from build123d import *

# Parameters (mm, degrees)
ESQUISSE1_W        = 1810
ESQUISSE1_H        = 1810
BOSS_EXTRU_1_DEPTH = 10
ESQUISSE2_W        = 1810
ESQUISSE2_H        = 1810
ESQUISSE2_W_2      = 1750
ESQUISSE2_H_2      = 1750
BOSS_EXTRU_2_DEPTH = 50
ESQUISSE3_W        = 1750
ESQUISSE3_H        = 30
BOSS_EXTRU_3_DEPTH = 50
ESQUISSE4_W        = 30
ESQUISSE4_H        = 1750
BOSS_EXTRU_4_DEPTH = 50
ESQUISSE5_W        = 1810
ESQUISSE5_H        = 1810
ESQUISSE5_W_2      = 1786
ESQUISSE5_H_2      = 1786
BOSS_EXTRU_5_DEPTH = 50


with BuildPart() as part:
    # Esquisse1 → Boss.-Extru.1 (new body)
    with BuildSketch(Plane(origin=(0, 0, 0), x_dir=(1, 0, 0), z_dir=(0, 1, 0))):
        Rectangle(ESQUISSE1_W, ESQUISSE1_H)
    extrude(amount=BOSS_EXTRU_1_DEPTH)

    # Esquisse2 → Boss.-Extru.2 (add)
    with BuildSketch(Plane(origin=(0, 0, 0), x_dir=(-1, 0, 0), z_dir=(0, -1, 0))):
        Rectangle(ESQUISSE2_W, ESQUISSE2_H)
        Rectangle(ESQUISSE2_W_2, ESQUISSE2_H_2, mode=Mode.SUBTRACT)
    extrude(amount=BOSS_EXTRU_2_DEPTH)

    # Esquisse3 → Boss.-Extru.3 (add)
    with BuildSketch(Plane(origin=(0, 0, 0), x_dir=(-1, 0, 0), z_dir=(0, -1, 0))):
        with Locations((0, -290)):
            Rectangle(ESQUISSE3_W, ESQUISSE3_H)
        with Locations((0, 290)):
            Rectangle(ESQUISSE3_W, ESQUISSE3_H)
    extrude(amount=BOSS_EXTRU_3_DEPTH)

    # Esquisse4 → Boss.-Extru.4 (add)
    with BuildSketch(Plane(origin=(0, 0, 0), x_dir=(-1, 0, 0), z_dir=(0, -1, 0))):
        with Locations((320, 0)):
            Rectangle(ESQUISSE4_W, ESQUISSE4_H)
        with Locations((-320, 0)):
            Rectangle(ESQUISSE4_W, ESQUISSE4_H)
    extrude(amount=BOSS_EXTRU_4_DEPTH)

    # Esquisse5 → Boss.-Extru.5 (add)
    with BuildSketch(Plane(origin=(0, 10, 0), x_dir=(1, 0, 0), z_dir=(0, 1, 0))):
        Rectangle(ESQUISSE5_W, ESQUISSE5_H)
        Rectangle(ESQUISSE5_W_2, ESQUISSE5_H_2, mode=Mode.SUBTRACT)
    extrude(amount=BOSS_EXTRU_5_DEPTH)


solid = part.part
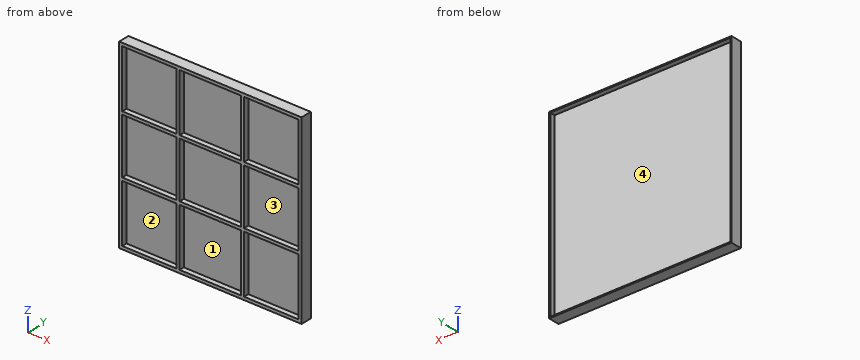
Check sheet for the modelled part. Datum: model origin and axes. Units: mm. Face numbers are marked on the shaded views. A direction names the side the tool comes from. Give positions to 0.01 mm unless a question says otherwise; leave off trailing zeros. Loops run counter-clockwise (first coordinate to the right, second up) from the corner with the lowest first, then second, coordinate; pieces in that order, holes last. Notation, with made-up numbers: M 1,-39 L 19,-39 A23 ccw 19,-11 Z; hole C 17,-33.5 d10. An arc over 180 degrees is marked long. Return JSON: item names as keys, results as strings. Group by question number.
1. Go/stop test with a flat-tipped pin: pin 1 (1.5 mm diameter, centred on x = 240, z = 129, fed in from -Y). Record where the tip stops, or that it passes through.
2. Cross-section at C-C on x = 373. Record the boundary of the cut face in (y, z), plus the area to 3 significant figures.
3. Tool access check on the marked faces 3 and 4. Record the directions out of +Z, -Z, +X, -X, +Y, -Y that give a thin tool (end or side, any length) a straight path to the whole face; none if there is none.
4. Mould release check, pull along Z, two halves, no side actions. Record for the marked faces 1 and 2: released by +Z, released by -Z, zero draft, split by the parting line, or undercut.
5. Cross-section at B-B on z = 773.5. Record the boundary of the cut face in (x, y), plus the area to 3 significant figures.
6. Cross-section at A-A on y = 34. Record the boundary of the cut face in (x, z).
7. Thickness scan on L1, parallel to Z at x = 625.5, y = -24; L2, parallel to X at y = -6.5, z = 623; L3, parallel to X at y = 38.5, z = -620.5. Record the ranges inside material, lowest first.
Return value:
{
 "1": {"pin 1": "y = 0"},
 "2": {"outline": "M -50,-905 L 60,-905 L 60,-893 L 10,-893 L 10,893 L 60,893 L 60,905 L -50,905 L -50,875 L 0,875 L 0,305 L -50,305 L -50,275 L 0,275 L 0,-275 L -50,-275 L -50,-305 L 0,-305 L 0,-875 L -50,-875 Z", "area": "25,300 mm^2"},
 "3": {"face 3": "-Y", "face 4": "+Y"},
 "4": {"face 1": "undercut", "face 2": "undercut"},
 "5": {"outline": "M -905,-50 L -875,-50 L -875,0 L -335,0 L -335,-50 L -305,-50 L -305,0 L 305,0 L 305,-50 L 335,-50 L 335,0 L 875,0 L 875,-50 L 905,-50 L 905,60 L 893,60 L 893,10 L -893,10 L -893,60 L -905,60 Z", "area": "25,300 mm^2"},
 "6": {"outline": "M -905,-905 L 905,-905 L 905,905 L -905,905 Z; hole M -893,-893 L 893,-893 L 893,893 L -893,893 Z"},
 "7": {"L1": "-905 to -875, -305 to -275, 275 to 305, 875 to 905", "L2": "-905 to -875, -335 to -305, 305 to 335, 875 to 905", "L3": "-905 to -893, 893 to 905"}
}
